Can you work these out from the model? Positions are in its coordinate system, mm. A direction names the side the tool comes from. Give positions to 0.01 mm unless a question says otherwise; leave off trailing zeros. Order: outer loops, then holes, each group sorted by start corner. A loop starts at its lowest first (then second) coordinate and runs counter-clockwise, first axis right, second up. Notation, with made-up numbers: (-2.5, -23.5) -> (38.5, -23.5) arc R18 ccw to (38.5, 6.5) -> close; hole circle Ø11 at (49.25, 27.5). An arc over 180 degrees is marked (long way). Answer as a JSON object with one key per item and string values.
Autodesk Inventor part; units mm, degrees
ref_plane "YZ Plane" through (0, 0, 0) normal (1, 0, 0) x (0, 1, 0)
ref_plane "XZ Plane" through (0, 0, 0) normal (0, 1, 0) x (-1, 0, 0)
ref_plane "XY Plane" through (0, 0, 0) normal (0, 0, 1) x (1, 0, 0)
sketch "Esquisse1" plane through (0, 0, 0) normal (0, 1, 0) x (-1, 0, 0)
  line L0 (0, 0) -> (500, 0)
  line L1 (500, 0) -> (500, -600)
  line L2 (500, -600) -> (0, -600)
  line L3 (0, -600) -> (0, 0)
  dimension "d0" = 500
  dimension "d1" = 600
extrude "Extrusion1" add sketch "Esquisse1" along normal blind 1700
sketch "Esquisse3" plane through (0, 1700, 0) normal (0, 1, 0) x (1, 0, 0)
  line L0 (-500, 600) -> (-500, 0)
  line L1 (0, 600) -> (-500, 600)
  line L2 (-500, 13.2496) -> (0, 13.2496)
  line L3 (0, 13.2496) -> (0, 600)
  line L4 (0, 600) -> (-500, 600)
  line L5 (-500, 600) -> (-500, 13.2496)
  point P0 (0, 0)
extrude "Extrusion2" cut sketch "Esquisse3" against normal blind 790
sketch "Esquisse4" plane through (0, 910, 0) normal (0, 1, 0) x (1, 0, 0)
  line L0 (0, 13.2496) -> (-500, 13.2496)
  line L1 (0, 13.2496) -> (-10, 13.2496)
  line L2 (0, 600) -> (-500, 600)
  line L3 (-500, 600) -> (-490, 600)
  line L4 (-490, 600) -> (-490, 590)
  line L5 (-490, 590) -> (-10, 590)
  line L6 (-10, 590) -> (-10, 13.2496)
  line L7 (-10, 13.2496) -> (-490, 13.2496)
  line L8 (-490, 13.2496) -> (-490, 590)
  point P0 (0, 0)
  dimension "d7" = 10
  dimension "d8" = 10
  dimension "d9" = 10
extrude "Extrusion3" cut sketch "Esquisse4" against normal blind 800
sketch "Esquisse5" plane through (0, 0, 0) normal (1, 0, 0) x (0, 0, -1)
  line L0 (600, 0) -> (600, 910)
  line L1 (600, 910) -> (800, 910)
  line L2 (800, 910) -> (817.3648, 1008.4808)
  line L3 (0, 0) -> (0, 1700)
  line L4 (0, 1700) -> (490, 1700)
  arc A0 (490, 1700) -> (817.3648, 1008.4808) centre (1204.9924, 1615.2302) ccw
  line L5 (13.2496, 1700) -> (13.2496, 910)
  line L6 (13.2496, 1700) -> (13.2496, 910)
  line L7 (13.2496, 910) -> (590, 910)
  line L8 (800, 910) -> (13.2496, 910)
  dimension "d12" = 200
  dimension "d13" = 100
  dimension "d14" = 100
  dimension "d15" = 490
  dimension "d16" = 720
extrude "Extrusion4" add sketch "Esquisse5" against normal blind 10
sketch "Esquisse6" plane through (-500, 0, -600) normal (-1, 0, 0) x (0, 0, 1)
  line L0 (0, 0) -> (0, 910)
  line L1 (0, 910) -> (-200, 910)
  line L2 (0, 910) -> (-200, 910)
  line L3 (-200, 910) -> (-217.3648, 1008.4808)
  line L4 (586.7504, 910) -> (586.7504, 110)
  line L5 (0, 910) -> (586.7504, 910)
  line L6 (586.7504, 1700) -> (110, 1700)
  line L7 (586.7504, 910) -> (586.7504, 1700)
  line L8 (586.7504, 1700) -> (110, 1700)
  arc A0 (-217.3648, 1008.4808) -> (110, 1700) centre (-604.9924, 1615.2302) ccw
  point P0 (600, 0)
  dimension "d19" = 100
  dimension "d20" = 100
sketch "Esquisse7" plane through (-500, 0, -600) normal (-1, 0, 0) x (0, 0, 1)
  line L0 (586.7504, 1700) -> (110, 1700)
  line L1 (110, 1700) -> (586.7504, 1700)
  line L2 (0, 0) -> (0, 910)
  line L3 (586.7504, 910) -> (10, 910)
  line L4 (0, 910) -> (586.7504, 910)
  line L5 (586.7504, 910) -> (586.7504, 1700)
  line L6 (0, 910) -> (-200, 910)
  line L7 (0, 910) -> (-200, 910)
  line L8 (-217.3648, 1008.4808) -> (-200, 910)
  line L9 (-200, 910) -> (-217.3648, 1008.4808)
  point P0 (600, 0)
extrude "Extrusion5" add sketch "Esquisse6" against normal blind 10
ref_plane "Plan de construction1" through (0, 910, -800) normal (0, -1, 0) x (1, 0, 0)
sketch "Esquisse8" plane through (0, 910, -800) normal (0, -1, 0) x (1, 0, 0)
  line L0 (-10, 0) -> (-10, 200)
  line L1 (0, 200) -> (-500, 200)
  line L2 (-10, 0) -> (-490, 0)
  line L3 (-490, 0) -> (-490, 200)
  line L4 (-490, 200) -> (-10, 200)
  line L5 (-10, 200) -> (-10, 0)
  point P0 (0, 800)
  dimension "d23" = 480
extrude "Extrusion6" add sketch "Esquisse8" against normal blind 10
sketch "Esquisse9" plane through (-490, 1008.4808, -817.3648) normal (0, -0.1736, -0.9848) x (-1, 0, 0)
  line L0 (-480, 541.3803) -> (-480, -1024.464)
  line L1 (0, -90.1519) -> (0, -100)
  line L2 (-480, -2.3513) -> (0, -2.3513)
  line L3 (0, -2.3513) -> (0, -90.1519)
  line L4 (0, -90.1519) -> (-480, -90.1519)
  line L5 (-480, -90.1519) -> (-480, -2.3513)
  point P0 (-490, -1135.0936)
extrude "Extrusion7" add sketch "Esquisse9" against normal blind 10
sketch "Esquisse10" plane through (0, 1700, 0) normal (0, 1, 0) x (1, 0, 0)
  point P0 (0, 0)
sketch "Esquisse11" plane through (0, 1700, 0) normal (0, 1, 0) x (1, 0, 0)
  line L0 (-500, 490) -> (-490, 490)
  line L1 (-490, 490) -> (-490, 10)
  line L2 (-490, 13.2496) -> (-490, 590)
  line L3 (-10, 590) -> (-10, 13.2496)
  line L4 (-10, 13.2496) -> (-490, 13.2496)
  line L5 (-10, 490) -> (-490, 490)
  line L6 (-490, 490) -> (-490, 13.2496)
  line L7 (-490, 13.2496) -> (-10, 13.2496)
  line L8 (-10, 13.2496) -> (-10, 490)
  point P0 (0, 0)
  dimension "d28" = 480
extrude "Extrusion8" add sketch "Esquisse11" against normal blind 10
sketch "Esquisse13" plane through (-490, 1006.1652, -816.9565) normal (0, 0.9848, -0.1736) x (1, 0, 0)
  line L0 (480, -10) -> (0, -10)
  line L1 (480, -10) -> (0, -10)
  line L2 (0, -10) -> (0, -210)
  line L3 (0, -210) -> (480, -210)
  line L4 (480, -210) -> (480, -10)
  point P0 (490, -629.8264)
  dimension "d33" = 480
  dimension "d34" = 200
extrude "Extrusion9" add sketch "Esquisse13" against normal blind 10
equation "\"RayonPli\" = Epaisseur"
equation "\"LargeurGrugeage\" = Epaisseur"
equation "\"ProfondeurGrugeage\" = 0.5 * Epaisseur"
equation "\"TailleGrugeage\" = 4 * Epaisseur"
equation "\"RestesMinimum\" = 2 * Epaisseur"
equation "\"Rayondetransition\" = RayonPli"
equation "\"TailleRayonJacobi\" = RayonPli"
equation "\"TailleJeu\" = Epaisseur"
1. Please list where these lines run through material, in increasing order: L1, parallel to Y at x = -443, z = -129.5; L2, parallel to X at y = 1229, z = -124; L3, parallel to Z at x = -260, y = 359.
Worked answers:
{"L1": "0 to 110, 1690 to 1700", "L2": "-500 to -490, -10 to 0", "L3": "-600 to -590, -13.25 to 0"}
2. For faces 1 (the face through (-253, 910, -699)), 2 (the face through (-253, 911, -13.25)), 3 (the face through (-253, 1690, -255)), 4 (the face through (-253, 516, -590)), which set-ups out of +Z, -Z, +X, -X, +Y, -Y let a thin tool reach every point of the face, with its end or its side?
Worked answers:
{"face 1": "-Z, +X, -X, -Y", "face 2": "none", "face 3": "-Z", "face 4": "+Y"}
3. If we section it at D-D on y = 1371: Please give me the cut outline in (x, z), then the cut area to 3 significant figures.
Worked answers:
{"outline": "(-500, -527.68) -> (-490, -527.68) -> (-490, -13.25) -> (-10, -13.25) -> (-10, -527.68) -> (0, -527.68) -> (0, 0) -> (-500, 0) -> close", "area": "16,900 mm²"}
4. If we mould it in two halves opening along X, with no side actions, what happens to faces 5 (the face through (-253.36, 1025.023, -710.006)), 6 (the face through (-246.64, 963.54, -809.44)), 7 (the face through (0, 862, -312)), 8 (the face through (-500, 862, -324))? For each: +X half, -X half, draft (parallel to the pull), parting line (faces both ways), or undercut.
Worked answers:
{"face 5": "undercut", "face 6": "draft", "face 7": "+X half", "face 8": "-X half"}
5. If we section it at A-A on y = 711: Please give me the cut outline in (x, z), then the cut area to 3 significant figures.
Worked answers:
{"outline": "(-500, -600) -> (0, -600) -> (0, 0) -> (-500, 0) -> close; hole (-490, -590) -> (-10, -590) -> (-10, -13.25) -> (-490, -13.25) -> close", "area": "23,200 mm²"}
6. If we section it at C-C on z = -362.5: Please give me the cut outline in (x, y).
Worked answers:
{"outline": "(-500, 0) -> (0, 0) -> (0, 1700) -> (-500, 1700) -> close; hole (-490, 110) -> (-10, 110) -> (-10, 1690) -> (-490, 1690) -> close"}
7. Will these pins go through, and if not, where does the flat tip stop? pin 1 Ø12 at (x, z) = (-85.5, -514) entering from +Y; pin 2 Ø1.5 at (x, y) = (-348, 1141) entering from -Z; pin 3 Ø8 at (x, y) = (-146.5, 915) entering from -Z.
Worked answers:
{"pin 1": "y = 110", "pin 2": "z = -13.25", "pin 3": "z = -800"}
